Geometry: see drawing. Coordinates: mm, zero at the bounding-box minimum. A direction names the side the tool comes from. Coordinates: 2 decimals unless noted, no trailing zeros.
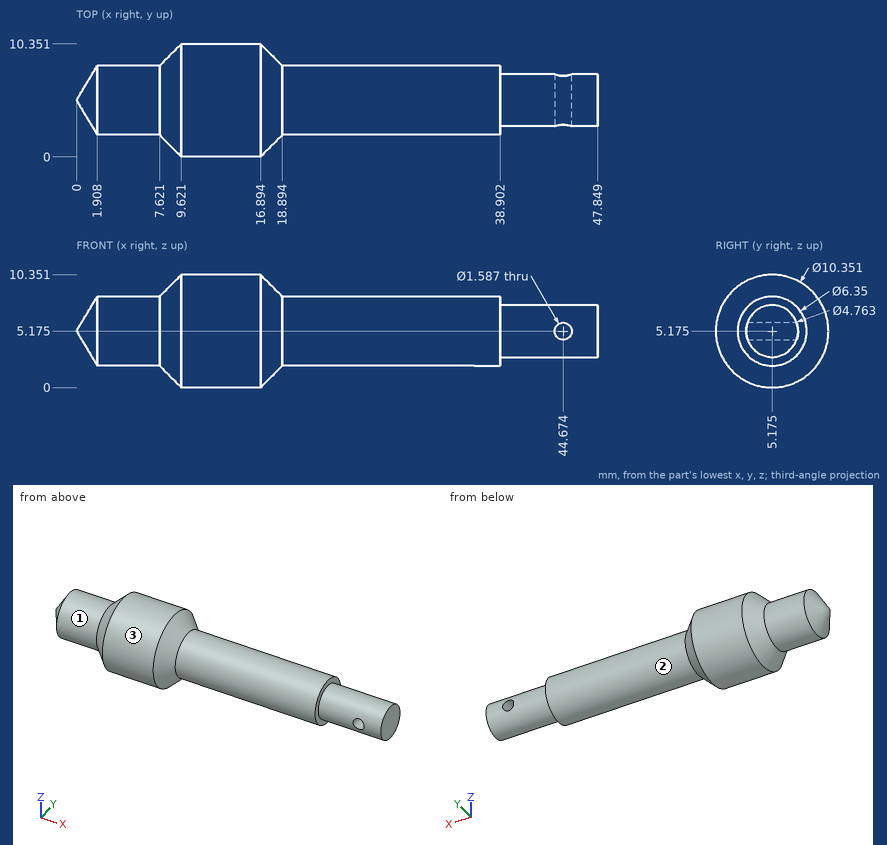
Item 1: Ray query, probe 1 along Y at (x, z) = (34, 5) (1 decimal); probe 2 along Z at (x, y) = (12, 5.5); probe 3 along X at (y, z) = (6.5, 5). Return the intervals inside material, ascending.
Response values:
probe 1: y = 2 to 8.3
probe 2: z = 0.01 to 10.34
probe 3: x = 0.8 to 43.9, 45.45 to 47.85
Item 2: Pin query (flat end, axial travel): pin 1 Ø6 at (x, y) = (33.5, 4.5) entering from +Z; pin 2 Ø3 at (x, y) = (40.5, 6.5) entering from -Z; pin 3 Ø3 at (x, z) = (41.5, 5) entering from +Y. Return the tip coordinate at first contact, or that it passes through.
Response values:
pin 1: stops at z = 8.35
pin 2: stops at z = 2.79
pin 3: stops at y = 7.56
Item 3: Access query for the marked faces 1, 2 and 3. Directions: +Z, -Z, +X, -X, +Y, -Y. A direction counts if a zero-diameter tool reaches every point of the face in a straight line with its end or side. Return the directions, or none.
Response values:
face 1: -X
face 2: +X
face 3: +X, -X
